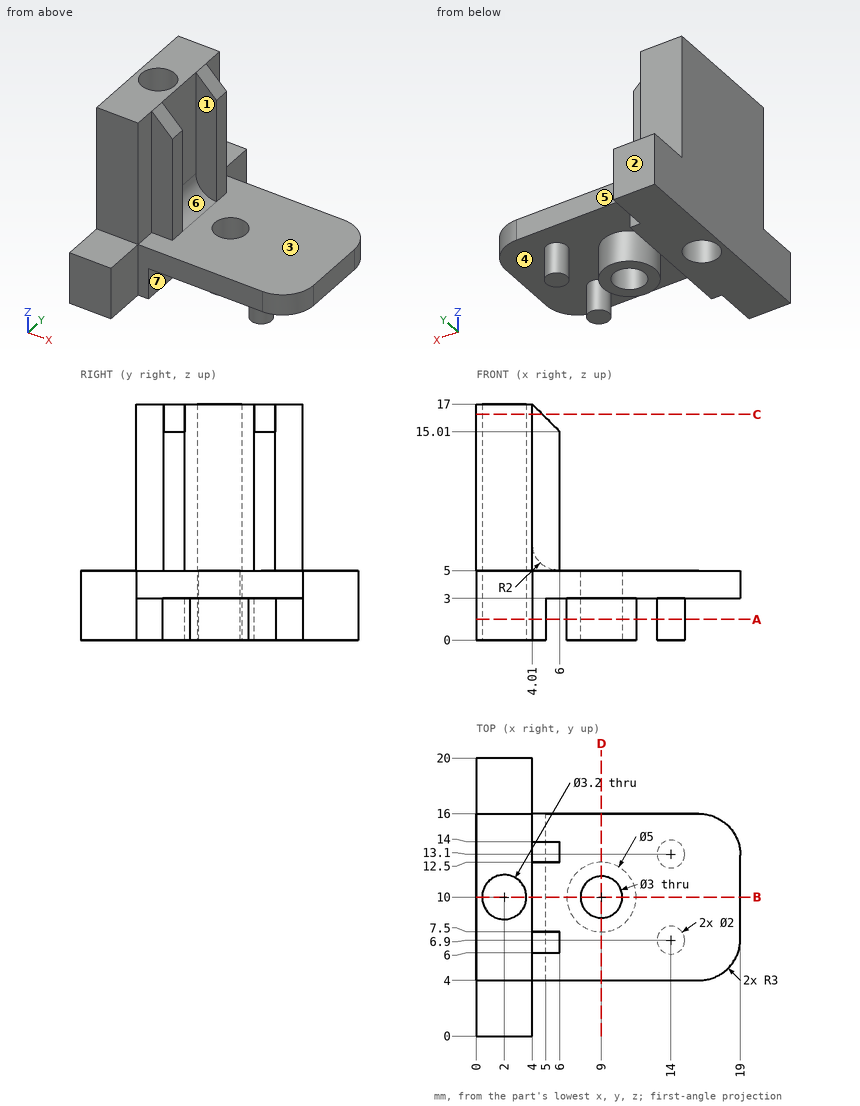
Here's the drawing with two shaded views (mm, measured from the low corner). I have some questions. A direction names the side the tool comes from. Coordinates: 2 decimals unless noted, no trailing zeros. Write each loop counter-clockwise with the first axis right and the second up, starting at its lowest first coordinate (ties: lowest second). Pieces come first, ordered by that corner, then holes. Notation, with made-up numbers: (53.5, -17.75) -> (64.5, -17.75) arc R23 ccw to (64.5, 13.25) -> close; hole circle Ø8 at (-0.75, 58.25). An arc over 180 degrees is marked (long way). One line per question, with ' | ' between items. Start each with the question number.
1. If we section it at C-C (z = 16.25): Please give me the cut outline in (x, y).
2. If we section it at B-B (y = 10): Please give me the cut outline in (x, z).
3. Will these pins go through, and if not, where does the flat tip stop? P1, Ø1.5, axis at x = 3, z = 7, coming from the +Y side; P2, Ø2, axis at x = 6.5, y = 7.5, coming from the -Z side; P3, Ø2, axis at x = 2, y = 1, coming from the +Z side.
4. Please list where these lines run through material, in increasing order: line 1 along Y through (x, z) = (9, 4.05); line 2 along Y through (x, z) = (2, 6.75); line 3 along Z through (x, y) = (15.25, 14.75).
5. Thinking about a two-plate mould opening in Y: for the marked faces 1, 2 and 3, which applies, pulls with the +Y half, pulls with the -Y half, needs draft (parallel to the pull), parting line crosses it, or undercut?
6. For the marked faces 4, 5, 6 and 7, which set-ups out of +Z, -Z, +X, -X, +Y, -Y let a thin tool reach every point of the face, with its end or its side?
7. If we section it at A-A (z = 1.5): Please give me the cut outline in (x, y).
8. If we section it at D-D (x = 9): Please give me the cut outline in (y, z), and give its area (3 significant figures).
Return value:
1) outline: (0, 4) -> (4, 4) -> (4, 6) -> (4.76, 6) -> (4.76, 7.5) -> (4, 7.5) -> (4, 12.5) -> (4.76, 12.5) -> (4.76, 14) -> (4, 14) -> (4, 16) -> (0, 16) -> close; hole circle Ø3.2 at (2, 10)
2) outline: (0, 0) -> (0.4, 0) -> (0.4, 17) -> (0, 17) -> close; (3.6, 0) -> (5, 0) -> (5, 3) -> (6.5, 3) -> (6.5, 0) -> (7.5, 0) -> (7.5, 5) -> (6, 5) arc R2 cw to (4, 7) -> (4, 17) -> (3.6, 17) -> close; (10.5, 0) -> (11.5, 0) -> (11.5, 3) -> (19, 3) -> (19, 5) -> (10.5, 5) -> close
3) P1: stops at y = 16 | P2: stops at z = 3 | P3: stops at z = 5
4) line 1: y = 4 to 8.5, 11.5 to 16 | line 2: y = 4 to 8.4, 11.6 to 16 | line 3: z = 3 to 5
5) face 1: undercut | face 2: pulls with the +Y half | face 3: needs draft
6) face 4: -Z | face 5: +Z, -Z, +X, +Y | face 6: +Z, +X | face 7: -Z, +Y, -Y
7) outline: (0, 0) -> (4, 0) -> (4, 4) -> (5, 4) -> (5, 16) -> (4, 16) -> (4, 20) -> (0, 20) -> close; circle Ø5 at (9, 10); circle Ø2 at (14, 6.9); circle Ø2 at (14, 13.1); hole circle Ø3.2 at (2, 10); hole circle Ø3 at (9, 10)
8) outline: (4, 3) -> (7.5, 3) -> (7.5, 0) -> (8.5, 0) -> (8.5, 5) -> (4, 5) -> close; (11.5, 0) -> (12.5, 0) -> (12.5, 3) -> (16, 3) -> (16, 5) -> (11.5, 5) -> close | area: 24.0 mm²
